from build123d import *

# Parameters (mm, degrees)
SKETCH1_R           = 73.025
SKETCH1_R_2         = 38.1
BOSS_EXTRUDE1_DEPTH = 15.875
SKETCH2_R           = 2.97688
CUT_EXTRUDE1_DEPTH  = 16.875
CIRPATTERN1_COUNT   = 16
SKETCH3_R           = 52.4383
SKETCH3_R_2         = 49.7967
CUT_EXTRUDE2_DEPTH  = 1.3208


with BuildPart() as part:
    # Sketch1 → Boss-Extrude1 (new body)
    with BuildSketch(Plane(origin=(0, 0, 0), x_dir=(1, 0, 0), z_dir=(0, 1, 0))):
        Circle(SKETCH1_R)
        Circle(SKETCH1_R_2, mode=Mode.SUBTRACT)
    extrude(amount=BOSS_EXTRUDE1_DEPTH)

    # Sketch2 → Cut-Extrude1 (cut, through all)
    with BuildSketch(Plane(origin=(0, 15.875, 0), x_dir=(1, 0, 0), z_dir=(0, 1, 0))):
        with Locations((67.31, 0)):
            Circle(SKETCH2_R)
    cut_extrude1 = extrude(amount=-CUT_EXTRUDE1_DEPTH, mode=Mode.SUBTRACT)

    # CirPattern1: Cut-Extrude1 ×16 about axis
    cirpattern1_axis = Axis((0, 0, 0), (0, 1, 0))
    for i in range(1, CIRPATTERN1_COUNT):
        add(cut_extrude1.rotate(cirpattern1_axis, i * 360 / CIRPATTERN1_COUNT), mode=Mode.SUBTRACT)

    # Sketch3 → Cut-Extrude2 (cut)
    with BuildSketch(Plane(origin=(0, 15.875, 0), x_dir=(1, 0, 0), z_dir=(0, 1, 0))):
        Circle(SKETCH3_R)
        Circle(SKETCH3_R_2, mode=Mode.SUBTRACT)
    extrude(amount=-CUT_EXTRUDE2_DEPTH, mode=Mode.SUBTRACT)


solid = part.part
Part model, mm, in its own coordinate system. A direction names the side the tool comes from. Give positions to 0.01 mm unless a question says otherwise; leave off trailing zeros. Loops run counter-clockwise (first coordinate to the right, second up) from the corner with the lowest first, then second, coordinate; pieces in that order, holes last. Notation, with made-up numbers: M 21.5,69 L 26.5,69 A22 ccw 26.5,103 Z; hole C -2,-2.5 d9. An arc over 180 degrees is marked long. Put each result on its own line as item: value. Start each with the question number.
1) Saw through at D-D (y = 8.75). State how many separate pieces and enclosed holes the cut face has, then the cut area to 3 significant figures.
2) Flat gauge pins, fed straight in: pin 1 (5.5 mm diameter, centred on x = 47.6, z = 47.6, fed in from -Y); pin 2 (5 mm diameter, centred on x = 37.5, y = 2, fed in from +Z); pin 3 (8 mm diameter, centred on y = 11.5, z = -35.5, fed in from +X); pin 4 (1 mm diameter, centred on x = -44.5, y = 4.5, fed in from +Z). Where does each tip first touch, or does it go through?
3) Saw through at B-B (z = 0). List the corners of the cut face in (x, y) (3 decimals).
4) 3-axis set-ups, long thin cutter, end or side, ignore diameter. For faces 4 (the cylindrical face through (-64.625, 8.049, -24.052)), 5 (the flat face through (46.4, 14.554, 19.2)): which of +Z, -Z, +X, -X, +Y, -Y reach the whole face in a straight line?
5) Probe probe 1 along X at (y, z) = (9.75, 49.5); probe 2 along Z at (x, y) = (-13.5, 1.5); probe 3 along Z at (x, y) = (4, 5.5). List the from-to ranges inside material, lowest first.
6) Saw through at C-C (z = -35). List the corners of the cut face in (x, y) (3 decimals).
7) Pull direction Z, two halves, no side cores. Call faces 1 (the flat face through (-22, 15.875, -49)), 2 (the cylindrical face through (69.653, 7.826, -21.935)), 3 (the cylindrical face through (-65.163, 8.049, 25.757)): +Z half, -Z half, draft (parallel to the pull), parting line (faces both ways), or undercut.
8) Saw through at A-A (x = 0). List the corners of the cut face in (y, z) (3 decimals).
Numbers:
1. separate pieces: 1
1. enclosed holes: 17
1. area: 11,700 mm^2
2. pin 1: through
2. pin 2: z = 64.09
2. pin 3: x = 65.88
2. pin 4: z = 58.28
3. outline: M -73.025,0 L -70.287,0 L -70.287,15.875 L -73.025,15.875 Z; M -64.333,0 L -38.1,0 L -38.1,15.875 L -49.797,15.875 L -49.797,14.554 L -52.438,14.554 L -52.438,15.875 L -64.333,15.875 Z; M 38.1,0 L 64.333,0 L 64.333,15.875 L 52.438,15.875 L 52.438,14.554 L 49.797,14.554 L 49.797,15.875 L 38.1,15.875 Z; M 70.287,0 L 73.025,0 L 73.025,15.875 L 70.287,15.875 Z
4. face 4: +Y, -Y
4. face 5: +Y
5. probe 1: -53.69 to -49.88, -45.31 to 45.31, 49.88 to 53.69
5. probe 2: -71.77 to -35.63, 35.63 to 71.77
5. probe 3: -72.92 to -37.89, 37.89 to 72.92
6. outline: M -64.091,0 L -15.054,0 L -15.054,15.875 L -35.422,15.875 L -35.422,14.554 L -39.048,14.554 L -39.048,15.875 L -64.091,15.875 Z; M 15.054,0 L 64.091,0 L 64.091,15.875 L 39.048,15.875 L 39.048,14.554 L 35.422,14.554 L 35.422,15.875 L 15.054,15.875 Z
7. face 1: draft
7. face 2: parting line
7. face 3: undercut
8. outline: M 0,-73.025 L 15.875,-73.025 L 15.875,-70.287 L 0,-70.287 Z; M 0,-64.333 L 15.875,-64.333 L 15.875,-52.438 L 14.554,-52.438 L 14.554,-49.797 L 15.875,-49.797 L 15.875,-38.1 L 0,-38.1 Z; M 0,38.1 L 15.875,38.1 L 15.875,49.797 L 14.554,49.797 L 14.554,52.438 L 15.875,52.438 L 15.875,64.333 L 0,64.333 Z; M 0,70.287 L 15.875,70.287 L 15.875,73.025 L 0,73.025 Z
